```python
from build123d import *

# Parameters (mm, degrees)
F0_W      = 85.343997
F0_H      = 43.952162
F3_DEPTH  = 25.4
F1_W      = 4.267193
F1_H      = 32.43072
F1_W_2    = 4.693918
F1_H_2    = 33.284161
F4_DEPTH  = 25.4
F2_W      = 4.693918
F2_H      = 33.710879
F2_W_2    = 3.840477
F2_H_2    = 32.857437
F5_DEPTH  = 25.4
F6_W      = 3.840476
F6_H      = 48.646077
F6_W_2    = 4.693918
F6_H_2    = 51.206397
F7_DEPTH  = 25.4
F8_W      = 85.770724
F8_H      = 25.17648
F9_DEPTH  = 25.4
F10_W     = 85.912641
F10_H     = 34.937669
F11_DEPTH = 25.4


with BuildPart() as f3:
    # F0 (on Top) → F3 (new body)
    with BuildSketch(Plane.XY):
        with Locations((-3.30708, 5.97408)):
            Rectangle(F0_W, F0_H)
    extrude(amount=F3_DEPTH)

    # F1 (on Front) → F4 (join)
    with BuildSketch(Plane.XZ):
        with Locations((-43.845478, -16.002001)):
            Rectangle(F1_W, F1_H)
        with Locations((36.591239, -16.64208)):
            Rectangle(F1_W_2, F1_H_2)
    extrude(amount=F4_DEPTH)

    # F2 (on Front) → F5 (join)
    with BuildSketch(Plane.XZ):
        with Locations((36.484562, -16.642081)):
            Rectangle(F2_W, F2_H)
        with Locations((-43.952159, -16.21536)):
            Rectangle(F2_W_2, F2_H_2)
    extrude(amount=F5_DEPTH)

    # F6 (on Top) → F7 (join)
    with BuildSketch(Plane.XY):
        with Locations((-44.165522, 13.22832)):
            Rectangle(F6_W, F6_H)
        with Locations((36.484562, 14.08176)):
            Rectangle(F6_W_2, F6_H_2)
    extrude(amount=F7_DEPTH)

    # F8 (on Front) → F9 (join)
    with BuildSketch(Plane.XZ):
        with Locations((-2.88036, 12.58824)):
            Rectangle(F8_W, F8_H)
    extrude(amount=F9_DEPTH)

    # F10 (on Front) → F11 (join)
    with BuildSketch(Plane.XZ):
        with Locations((-3.794318, -17.468834)):
            Rectangle(F10_W, F10_H)
    extrude(amount=F11_DEPTH)


solid = f3.part
```
The model under review builds one solid part; all positions refer to its coordinate system, in mm. A direction names the side the tool comes from. Round coordinates to 2 decimals unless told otherwise and drop trailing zeros. Write each loop counter-clockwise with the first axis right and the second up, starting at its lowest first coordinate (ties: lowest second). Pieces come first, ordered by that corner, then holes. Notation, with made-up numbers: (24, 8.25) - (79, 8.25) arc R7 cw to (79, 12.25) - close; hole circle Ø9 at (-24.75, -6). An arc over 180 degrees is marked (long way). Use one line per item in the form item = value.
Q1. Consider section A-A (y = 32). State the section outline as (x, z) points, and give its area (3 significant figures).
Answer key:
outline = (-46.09, 0) - (-42.25, 0) - (-42.25, 25.4) - (-46.09, 25.4) - close; (34.14, 0) - (38.83, 0) - (38.83, 25.4) - (34.14, 25.4) - close
area = 217 mm2
Q2. Insertion check: pin 1 Ø12.5 at (y, z) = (17.5, 9) entering from -X; pin 2 Ø1.5 at (x, y) = (-1, 10.5) entering from -Z; pin 3 Ø1.5 at (y, z) = (-13.5, 18) entering from -X; pin 4 Ø12 at (y, z) = (7.5, -7.5) entering from -X. Each pin has a flat end and moves straight along its axis. Give the tip position at first contact, or say it passes through.
Answer key:
pin_1 = -46.09
pin_2 = 0
pin_3 = -45.98
pin_4 = through
Q3. Draft analysis for pull direction X (two halves, no side actions). For faces 1 (the flat face through (-42.245, 33, 13)), 2 (the flat face through (38.832, 34, 13)), 3 (the flat face through (36, 39.685, 13)), 4 (the flat face through (-46.751, -13, -18)), state which applies: +X half, -X half, draft (parallel to the pull), parting line (faces both ways), or undercut.
Answer key:
face_1 = undercut
face_2 = +X half
face_3 = draft
face_4 = -X half
Q4. Consider section C-C (z = -25.5). State the section outline as (x, y) points, and give its area (3 significant figures).
Answer key:
outline = (-46.75, -25.4) - (39.16, -25.4) - (39.16, 0) - (-46.75, 0) - close
area = 2,180 mm2
Q5. For line 1 (Z direction, x = 0, y = 16); line 2 (Y direction, x = -36, z = -2.5); line 3 (X direction, y = -21, z = -17), list the stretches that pass through material, from the lowest coordinate up. Write a range as [from, to].
Answer key:
line_1 = [0, 25.4]
line_2 = [-25.4, 0]
line_3 = [-46.75, 39.16]
Q6. Consider section B-B (x = -9.5). State the section outline as (y, z) points.
Answer key:
outline = (-25.4, -34.94) - (0, -34.94) - (0, 0) - (27.95, 0) - (27.95, 25.4) - (-16, 25.4) - (-16, 25.18) - (-25.4, 25.18) - close
Q7. Consider section D-D (y = 25). State the section outline as (x, z) points, and give its area (3 significant figures).
Answer key:
outline = (-46.09, 0) - (39.36, 0) - (39.36, 25.4) - (-46.09, 25.4) - close
area = 2,170 mm2
Q8. Tool access review of faces 5 (the flat face through (-4, 0, -17)), 6 (the flat face through (39.162, -13, -18)), 7 (the flat face through (-46.086, 13, 13)), 8 (the flat face through (-45.979, -14, 13)): name each direction out of +Z, -Z, +X, -X, +Y, -Y from which nothing blocks a thin tool from reaching the whole face with its end or side.
Answer key:
face_5 = -Z, +X, -X, +Y
face_6 = -Z, +X, +Y, -Y
face_7 = +Z, -X, +Y, -Y
face_8 = +Z, -X, -Y
